```python
from build123d import *

# Parameters (mm, degrees)
F2_R     = 12.030304
F3_DEPTH = 23.7


with BuildPart() as f1:
    # F0 (on Front) → F1 (revolve)
    with BuildSketch(Plane.XZ):
        Polygon((21.5, 15.483735), (3, 23.423815), (7, 0), (7, 12.614677), (12, 12.614677), (12, 0), (21.5, 0), align=None)
    revolve(axis=Axis((0, 0, 20), (0, 0, 1)))

    # F2 (on Top) → F3 (join)
    with BuildSketch(Plane.XY):
        with BuildLine():
            Line((16.699362, 21.699362), (-16.699362, 21.699362))
            ThreePointArc((-16.699362, 21.699362), (-20.234895, 20.234895), (-21.699362, 16.699362))
            Line((-21.699362, 16.699362), (-21.699362, -16.699362))
            ThreePointArc((-21.699362, -16.699362), (-20.234895, -20.234895), (-16.699362, -21.699362))
            Line((-16.699362, -21.699362), (16.699362, -21.699362))
            ThreePointArc((16.699362, -21.699362), (20.234895, -20.234895), (21.699362, -16.699362))
            Line((21.699362, -16.699362), (21.699362, 16.699362))
            ThreePointArc((21.699362, 16.699362), (20.234895, 20.234895), (16.699362, 21.699362))
        make_face()
        Circle(F2_R, mode=Mode.SUBTRACT)
    extrude(amount=F3_DEPTH)


solid = f1.part
```
CAD build for the part. Positions are in the model's coordinates, mm. A direction names the side the tool comes from. Give positions to 0.01 mm unless a question says otherwise; leave off trailing zeros. Order: outer loops, then holes, each group sorted by start corner. A loop starts at its lowest first (then second) coordinate and runs counter-clockwise, first axis right, second up.
(1) Drill centre lines: L1, parallel to Y at x = 0, z = 21.7; L2, parallel to X at y = 0, z = 21.65; L3, parallel to Y at x = 0, z = 22.8. Where is each one in solid material? Low to high.
(2) Saw through at A-A, the plane y = 0. Give the cut face in (x, z).
(3) Saw through at C-C, the plane z = 22. Give the cut face in (x, y).
(4) Saw through at D-D, the plane z = 16.25. Give the cut face in (x, y).
(5) Mould opens along Y. For faces 1 (the cylindrical face through (-20.2, 20.27, 11.68)), 2 (the cylindrical face through (11.475, 3.614, 21.595)), 3 (the conical face through (-2.729, -2.092, 23.236)), 4 (the cylindrical face through (20.2, -20.27, 11.68)) say: released by +Y, released by -Y, zero draft, split by the parting line, or undercut.
(6) Flat gauge pins, fed straight in: pin 1 (14.5 mm diameter, centred on x = 0, y = 0, fed in from +Z); pin 2 (1 mm diameter, centred on x = 8.5, y = -1.5, fed in from -Z). Where does each tip first touch, or does it go through?
(7) Tool access for faces 5 (the cylindrical face through (-11.99, 0.53, 6.22)), 6 (the flat face through (21.699, 0, 12)): list every direction of +Z, -Z, +X, -X, +Y, -Y with a clear straight run to the whole face (end or side of a thin tool).
Results found:
1. L1: y = -21.7 to -12.03, -7.02 to -3.29, 3.29 to 7.02, 12.03 to 21.7
1. L2: x = -21.7 to -12.03, -7.13 to -3.3, 3.3 to 7.13, 12.03 to 21.7
1. L3: y = -21.7 to -12.03, -4.45 to -3.11, 3.11 to 4.45, 12.03 to 21.7
2. outline: (-21.7, 0) - (-12, 0) - (-12, 12.61) - (-7, 12.61) - (-7, 0) - (-3, 23.42) - (-12.03, 19.55) - (-12.03, 23.7) - (-21.7, 23.7) - close; (3, 23.42) - (7, 0) - (7, 12.61) - (12, 12.61) - (12, 0) - (21.7, 0) - (21.7, 23.7) - (12.03, 23.7) - (12.03, 19.55) - close
3. outline: (-21.7, -16.7) arc R5 ccw to (-16.7, -21.7) - (16.7, -21.7) arc R5 ccw to (21.7, -16.7) - (21.7, 16.7) arc R5 ccw to (16.7, 21.7) - (-16.7, 21.7) arc R5 ccw to (-21.7, 16.7) - close; circle Ø12.63 at (0, 0); hole circle Ø24.06 at (0, 0); hole circle Ø6.49 at (0, 0)
4. outline: (-21.7, -16.7) arc R5 ccw to (-16.7, -21.7) - (16.7, -21.7) arc R5 ccw to (21.7, -16.7) - (21.7, 16.7) arc R5 ccw to (16.7, 21.7) - (-16.7, 21.7) arc R5 ccw to (-21.7, 16.7) - close; hole circle Ø8.45 at (0, 0)
5. face 1: released by +Y
5. face 2: undercut
5. face 3: undercut
5. face 4: released by -Y
6. pin 1: stops at z = 23.42
6. pin 2: stops at z = 12.61
7. face 5: -Z
7. face 6: +Z, -Z, +X, +Y, -Y
